Geometry check sheet. Reference: the model listing, model coordinates, mm. Face numbers are marked on the shaded views. Give positions to 0.01 mm unless a question says otherwise; leave off trailing zeros.
1. Material ranges on L1, parallel to Z at x = -2, y = 21.25; L2, parallel to Y at x = 0, z = 74.6; L3, parallel to Y at x = 0, z = 74, recorded low to high.
2. Go/stop test with a flat-tipped pin: pin 1 Ø15.5 at (x, y) = (-1, 15) entering from +Z. Record where the tip stops, or that it passes through.
3. Release check for a two-part mould opening along Y. For the marked faces 1, 2, 3 and 4 record: +Y half, -Y half, draft (parallel to the pull), parting line (faces both ways), or undercut.
from build123d import *

# Parameters (mm, degrees)
SKETCH2_W           = 50
SKETCH2_H           = 150
BOSS_EXTRUDE1_DEPTH = 30
FILLET1_R           = 2
SKETCH3_R           = 9.81775282
CUT_EXTRUDE1_DEPTH  = 0.5


with BuildPart() as part:
    # Sketch2 → Boss-Extrude1 (new body)
    with BuildSketch(Plane(origin=(0, 0, 0), x_dir=(1, 0, 0), z_dir=(0, 1, 0))):
        Rectangle(SKETCH2_W, SKETCH2_H)
    extrude(amount=BOSS_EXTRUDE1_DEPTH)

    # Fillet1
    fillet1_edges = [part.edges().sort_by_distance(p)[0] for p in [
        (-25, 30, 0),
        (0, 30, 75),
        (25, 30, 0),
        (0, 0, 75),
        (-25, 0, 0),
        (0, 0, -75),
        (25, 0, 0),
        (25, 15, 75),
        (-25, 15, 75),
        (-25, 15, -75),
        (25, 15, -75),
        (0, 30, -75),
    ]]
    fillet(fillet1_edges, radius=FILLET1_R)

    # Sketch3 → Cut-Extrude1 (cut)
    with BuildSketch(Plane.XY.offset(75)):
        with Locations((0, 15)):
            Circle(SKETCH3_R)
    extrude(amount=-CUT_EXTRUDE1_DEPTH, mode=Mode.SUBTRACT)


solid = part.part
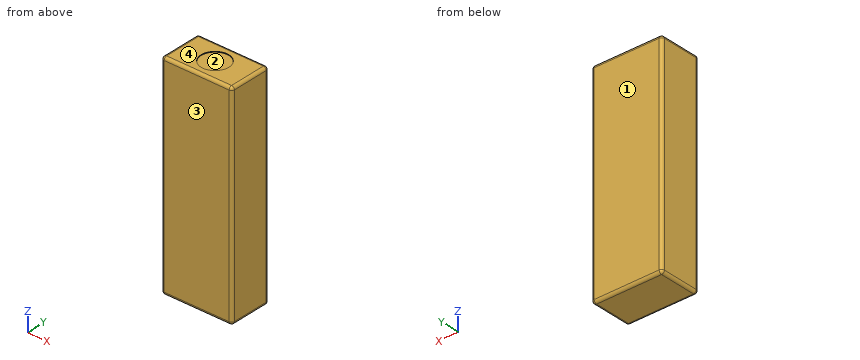
Result:
1. L1: z = -75 to 74.5
1. L2: y = 0.8 to 5.18, 24.82 to 29.2
1. L3: y = 0.27 to 29.73
2. pin 1: stops at z = 74.5
3. face 1: +Y half
3. face 2: undercut
3. face 3: -Y half
3. face 4: draft
